Input: part model. Units: mm. Frame: model coordinates. Face numbers are marked on the shaded views. A direction names the side the tool comes from. Coordinates: 2 decimals unless noted, no trailing zeros. Write each loop counter-clockwise with the first axis right and the second up, starting at its lowest first coordinate (ties: lowest second). Pieces come first, ordered by that corner, then holes. Notation, with made-up numbers: (52, -11) - (62, -11) arc R19 cw to (62, 21) - close; hole circle Ø4 at (5, 7.5). An arc over 180 degrees is marked (long way). Put each result on its own line as item: value. Start each with the question number.
1. Cut plane A-A, the plane z = 0. Return loops of the section in (x, y), and give its area (3 significant figures).
2. Line query: line 1 (X direction, y = -4.25, z = 8.75); line 2 (Y direction, x = 26.35, z = 0); line 3 (Z direction, x = 6.5, y = 0). Output: solid intervals per line, ascending.
3. Pull-direction query (Y, two-part tool) for the marked faces 1, 2 and 3; classes: released by +Y, released by -Y, zero draft, split by the parting line, or undercut.
4. Pin query (flat end, axial travel): pin 1 (10 mm diameter, centred on x = 7.5, z = -11, fed in from +Y); pin 2 (14 mm diameter, centred on y = 1, z = 1.5, fed in from +X); pin 3 (10 mm diameter, centred on x = 16, z = -8.5, fed in from +Y); pin 4 (5 mm diameter, centred on x = 24, y = -1, fed in from +Z). Return the tip coordinate at first contact, or that it passes through.
5. Access query for the marked faces 4, 5, 6 and 7. Directions: +Z, -Z, +X, -X, +Y, -Y. A direction counts if a zero-diameter tool reaches every point of the face in a straight line with its end or side. Return the directions, or none.
6. Cut plane B-B, the plane y = 11. Return loops of the section in (x, z).
7. Cut plane C-C, the plane x = 8. Return loops of the section in (y, z), and give its area (3 significant figures).
Autodesk Inventor part; units mm, degrees
ref_plane "YZ Plane" through (0, 0, 0) normal (1, 0, 0) x (0, 1, 0)
ref_plane "XZ Plane" through (0, 0, 0) normal (0, 1, 0) x (-1, 0, 0)
ref_plane "XY Plane" through (0, 0, 0) normal (0, 0, 1) x (1, 0, 0)
sketch "Sketch1" plane through (0, 0, 0) normal (1, 0, 0) x (0, 1, 0)
  circle A0 centre (0, 0) radius 9.144
  line L0 (0, 0) -> (9.144, 0)
  line L1 (9.144, 0) -> (9.144, -9.144)
  line L2 (9.144, -9.144) -> (0, -9.144)
  line L3 (0, -9.144) -> (0, 0)
  line L4 (0, 0) -> (9.144, 0)
  line L5 (9.144, 0) -> (9.144, 9.144)
  line L6 (9.144, 9.144) -> (0, 9.144)
  line L7 (0, 9.144) -> (0, 0)
  dimension "d0" = 18.288
extrude "Extrusion1" add sketch "Sketch1" along normal blind 13.97
sketch "Sketch5" plane through (13.97, 0, 0) normal (1, 0, 0) x (0, 0, -1)
  line L0 (9.144, 0) -> (9.144, 9.144)
  circle A0 centre (0, 0) radius 9.144
  line L1 (9.144, 9.144) -> (-9.144, 9.144)
  line L2 (-9.144, 9.144) -> (-9.144, 0)
  line L3 (-9.144, 0) -> (9.144, 0)
  line L4 (9.144, 0) -> (9.144, 9.144)
  point P0 (0, 9.144)
extrude "Extrusion5" cut sketch "Sketch5" against normal blind 25.4 contours A0 L1 L0 | L2 L1 A0
sketch "Sketch6" plane through (13.97, 0, 0) normal (1, 0, 0) x (0, 0, -1)
  circle A0 centre (0, 0) radius 3.2131
  dimension "d12" = 6.4262
extrude "Extrusion6" cut sketch "Sketch6" against normal blind 25.4
sketch "Sketch7" plane through (0, 0, 0) normal (-1, 0, 0) x (0, 0, 1)
  point P0 (0, 0)
sketch "Sketch8" plane through (13.97, 0, 0) normal (1, 0, 0) x (0, 0, -1)
  circle A0 centre (0, 0) radius 13.97
  dimension "d15" = 27.94
extrude "Extrusion7" add sketch "Sketch8" along normal blind 3.81
sketch "Sketch9" plane through (0, 0, 0) normal (-1, 0, 0) x (0, 0, 1)
  circle A0 centre (0, 0) radius 13.97
extrude "Extrusion8" add sketch "Sketch9" along normal blind 3.81
sketch "Sketch10" plane through (17.78, 0, 0) normal (1, 0, 0) x (0, 0, -1)
  line L0 (6.35, 0) -> (6.35, 6.35)
  line L1 (6.35, 6.35) -> (0, 6.35)
  line L2 (6.35, 6.35) -> (-6.35, 6.35)
  line L3 (-6.35, 6.35) -> (-6.35, -6.35)
  line L4 (-6.35, -6.35) -> (6.35, -6.35)
  line L5 (6.35, -6.35) -> (6.35, 6.35)
  point P0 (0, 0)
  dimension "d20" = 6.35
  dimension "d21" = 6.35
  dimension "d22" = 12.7
  dimension "d23" = 12.7
extrude "Extrusion9" add sketch "Sketch10" along normal blind 10.16
sketch "Sketch11" plane through (17.78, 6.35, 6.35) normal (0, 1, 0) x (1, 0, 0)
  line L0 (0, 12.7) -> (10.16, 12.7)
  line L1 (0, -7.62) -> (0, 20.32)
  line L2 (5.08, 3.1902) -> (5.08, 2.9362)
  line L3 (5.08, 9.8043) -> (8.054, 8.0873)
  line L4 (8.054, 8.0873) -> (8.054, 4.6532)
  line L5 (8.054, 4.6532) -> (5.08, 2.9362)
  line L6 (5.08, 2.9362) -> (2.106, 4.6532)
  line L7 (2.106, 4.6532) -> (2.106, 8.0873)
  line L8 (2.106, 8.0873) -> (5.08, 9.8043)
  point P0 (-17.78, 6.35)
  point P1 (-17.78, 7.62)
  point P2 (15.24, 15.24)
extrude "Extrusion10" cut sketch "Sketch11" against normal blind 25.4
sketch "Sketch12" plane through (27.94, 0, 0) normal (1, 0, 0) x (0, 0, -1)
  circle A0 centre (0, 0) radius 3.2131
extrude "Extrusion11" cut sketch "Sketch12" against normal blind 50.8
properties part number "230307 Bottom Pulley Adjusted"
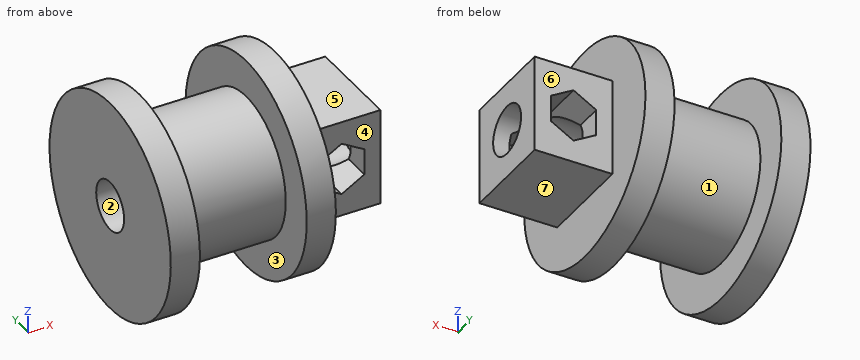
Report:
1. outline: (-3.81, -13.97) - (0, -13.97) - (0, -9.14) - (13.97, -9.14) - (13.97, -13.97) - (17.78, -13.97) - (17.78, -6.35) - (19.89, -6.35) - (19.89, -3.21) - (-3.81, -3.21) - close; (-3.81, 3.21) - (19.89, 3.21) - (19.89, 6.35) - (17.78, 6.35) - (17.78, 13.97) - (13.97, 13.97) - (13.97, 9.14) - (0, 9.14) - (0, 13.97) - (-3.81, 13.97) - close; (25.83, -6.35) - (27.94, -6.35) - (27.94, -3.21) - (25.83, -3.21) - close; (25.83, 3.21) - (27.94, 3.21) - (27.94, 6.35) - (25.83, 6.35) - close
1. area: 356 mm^2
2. line 1: x = -3.81 to 0, 13.97 to 17.78
2. line 2: y = -6.35 to -3.21, 3.21 to 6.35
2. line 3: z = -9.14 to -3.21, 3.21 to 9.14
3. face 1: split by the parting line
3. face 2: undercut
3. face 3: zero draft
4. pin 1: stops at y = 6.9
4. pin 2: stops at x = 27.94
4. pin 3: stops at y = 13.52
4. pin 4: stops at z = 6.35
5. face 4: +Z, -Z, +X, -Y
5. face 5: +Z, +X, +Y, -Y
5. face 6: +Z, -Z, +X, +Y
5. face 7: -Z, +X, +Y, -Y
6. outline: (-3.81, -8.61) - (0, -8.61) - (0, 8.61) - (-3.81, 8.61) - close; (13.97, -8.61) - (17.78, -8.61) - (17.78, 8.61) - (13.97, 8.61) - close
7. outline: circle Ø18.29 at (0, 0); hole circle Ø6.43 at (0, 0)
7. area: 230 mm^2
